Autodesk Inventor part; units mm, degrees
ref_plane "YZ Plane" through (0, 0, 0) normal (1, 0, 0) x (0, 1, 0)
ref_plane "XZ Plane" through (0, 0, 0) normal (0, 1, 0) x (-1, 0, 0)
ref_plane "XY Plane" through (0, 0, 0) normal (0, 0, 1) x (1, 0, 0)
sketch "Sketch1" plane through (0, 0, 0) normal (0, 0, 1) x (1, 0, 0)
  line L0 (0, 0) -> (80, 0)
  line L1 (0, 80) -> (0, 0)
  line L2 (40, 0) -> (160, 0) construction
  line L3 (0, 80) -> (80, 231.8222)
  line L4 (80, 231.8222) -> (142.1166, 231.8222)
  arc A0 (142.1166, 231.8222) -> (80, 0) centre (367.4632, 47.2076) ccw
  dimension "d2" = 240
  dimension "d4" = 80
extrude "Extrusion1" add sketch "Sketch1" along normal blind 20
chamfer "Chamfer1" distance 30 angle 45 1 edges at (0, 80, 10)
sketch "Sketch2" plane through (80, 231.8222, 0) normal (0, 1, 0) x (1, 0, 0)
  line L0 (62.1166, 0) -> (62.1166, -20)
  line L1 (62.1166, -10) -> (32.1166, -10)
  circle A0 centre (32.1166, -10) radius 5
  point P0 (-80, 0)
  dimension "d10" = 30
  dimension "d11" = 10
extrude "Extrusion2" cut sketch "Sketch2" against normal blind 10
properties part number "Base_Aerofoil"
Work out the finished part from the listing and answer in its coordinate system (mm). Round coordinates to 2 decimals unless told otherwise and drop trailing zeros. Write each loop counter-clockwise with the first axis right and the second up, starting at its lowest first coordinate (ties: lowest second). Pieces come first, ordered by that corner, then holes. Notation, with made-up numbers: (30, 78) - (51, 78) arc R4 cw to (51, 82) - close; hole circle Ø10 at (35.25, 65). An arc over 180 degrees is marked (long way). Return JSON: item names as keys, results as strings. Group by question number.
Q1. The part is cut by section D-D on x = 18. Write down the section's boundary in (y, z), then the cut area to 3 significant figures.
Q2. The part is cut by section B-B on x = 111. Write down the section's boundary in (y, z), then the cut area to 3 significant figures.
Q3. The part is cut by section A-A on z = 10. Write down the section's boundary in (x, y).
Q4. Find the intervals of material crossed by L1, parallel to X at y = 224.5, z = 10; L2, parallel to X at y = 227.5, z = 10; L3, parallel to X at y = 174, z = 12.25, in increasing order.
Q5. The part is cut by section C-C on y = 62.5. Write down the section's boundary in (x, z).
Q6. The mould has two halves that part along X. Classify faces 1 (the flat face through (7.1, 78.7, 10.1)), 2 (the flat face through (39, 0, 10)), 3 (the cylindrical face through (107.12, 226.89, 9.78)), 4 (the flat face through (112, 221.822, 10)): released by +X, released by -X, zero draft, split by the parting line, or undercut.
Q7. Each of these flat-tipped pins is pushed along its axis until it touches: pin 1 Ø11 at (x, z) = (111, 11.5) entering from +Y; pin 2 Ø8 at (y, z) = (143, 5) entering from -X; pin 3 Ø10 at (x, z) = (30, 2.5) entering from +Y; pin 4 Ø12 at (y, z) = (137.5, 14.5) entering from -X. Where does it stop, or does it pass through?
Solved:
{
 "1": {"outline": "(0, 0) - (114.16, 0) - (114.16, 20) - (0, 20) - close", "area": "2,280 mm²"},
 "2": {"outline": "(185.38, 0) - (231.82, 0) - (231.82, 5.13) - (221.82, 5.13) - (221.82, 14.87) - (231.82, 14.87) - (231.82, 20) - (185.38, 20) - close", "area": "831 mm²"},
 "3": {"outline": "(0, 0) - (80, 0) arc R291.31 cw to (142.12, 231.82) - (117.12, 231.82) - (117.12, 221.82) - (107.12, 221.82) - (107.12, 231.82) - (80, 231.82) - (13.99, 106.54) - (0, 50) - close"},
 "4": {"L1": "76.14 to 107.12, 117.12 to 136.31", "L2": "77.72 to 107.12, 117.12 to 138.64", "L3": "49.53 to 105.19"},
 "5": {"outline": "(3.09, 0) - (76.55, 0) - (76.55, 20) - (3.09, 20) - close"},
 "6": {"face 1": "released by -X", "face 2": "zero draft", "face 3": "undercut", "face 4": "undercut"},
 "7": {"pin 1": "y = 231.82", "pin 2": "x = 31.09", "pin 3": "y = 146.42", "pin 4": "x = 27.14"}
}
